from build123d import *

# Parameters (mm, degrees)
F0_W     = 431.8
F0_H     = 431.8
F1_DEPTH = 19.05
F3_DEPTH = 19.051
F5_DEPTH = 19.05
F7_DEPTH = 19.051
F9_DEPTH = 19.05


with BuildPart() as f1:
    # F0 (on Front) → F1 (new body)
    with BuildSketch(Plane.XZ):
        with Locations((215.9, 215.9)):
            Rectangle(F0_W, F0_H)
    extrude(amount=F1_DEPTH)

    # F2 (on face) → F3 (cut, through all)
    with BuildSketch(Plane.XZ.offset(19.05)):
        Polygon((177.8, 215.9), (50.8, 381), (50.8, 50.8), align=None)
        Polygon((381, 50.8), (381, 381), (254, 215.9), align=None)
    extrude(amount=-F3_DEPTH, mode=Mode.SUBTRACT)

    # F4 (on face) → F5 (join, through all)
    with BuildSketch(Plane.XZ.offset(19.05)):
        Polygon((0, 0), (0, 431.8), (-101.6, 914.4), (-152.4, 914.4), (-152.4, 0), align=None)
    extrude(amount=-F5_DEPTH)

    # F6 (on face) → F7 (cut, through all)
    with BuildSketch(Plane.XZ.offset(19.05)):
        Polygon((-101.6, 0), (-152.4, 914.4), (-152.4, 0), align=None)
    extrude(amount=-F7_DEPTH, mode=Mode.SUBTRACT)

    # F8 (on face) → F9 (join)
    with BuildSketch(Plane.XZ.offset(19.05)):
        Polygon((419.768421, 609.6), (-37.431579, 609.6), (0, 431.8), (101.6, 533.4), (343.568421, 533.4), align=None)
    extrude(amount=-F9_DEPTH)


solid = f1.part
Read the model definition and answer for the solid it produces. Units are mm, in the model's axes. A direction names the side the tool comes from. Give positions to 0.01 mm unless a question says otherwise; leave off trailing zeros. Write each loop counter-clockwise with the first axis right and the second up, starting at its lowest first coordinate (ties: lowest second). Pieces come first, ordered by that corner, then holes. Notation, with made-up numbers: (-14, -3.5) - (17, -3.5) arc R17 cw to (17, 24.5) - close; hole circle Ø2 at (15.5, 18). An arc over 180 degrees is marked (long way). Answer in a Markdown table with one row per item. Add a question column.
Item 1: Find the intervals of material crossed by L1, parallel to Z at x = 224, y = -17.25; L2, parallel to Z at x = 129, y = -15; L3, parallel to X at y = -12.25, z = 225, in increasing order.
Item 2: Section A-A, the plane x = 115.5 is taken. Write down the section's boundary in (y, z).
Item 3: Section D-D, the plane x = 13.5 is taken. Write down the section's boundary in (y, z).
Item 4: Determine the mould class of faces 1 (the face through (213, -9, 431.8)), 2 (the face through (115.19, -9.66, 297.29)), 3 (the face through (318.39, -9.66, 299.61)), 4 (the face through (50.1, -9.7, 481.9)) for opening direction X: pulls with the +X half, pulls with the -X half, needs draft (parallel to the pull), parting line crosses it, or undercut.
Item 5: A tool of negligible diameter and unlimited length cuts with its end or side. For faces 5 (the face through (316.61, -9.66, 134.51)), 6 (the face through (194, -10, 609.6)), 7 (the face through (381.14, -9.66, 570.97)), from which of +Z, -Z, +X, -X, +Y, -Y can it reach the whole face along a straight path? Write none if from no direction.
Item 6: Flat-ended cylindrical pins translate along their axes: P1, Ø5, axis at x = 320.5, z = 371.5, coming from the +Y side; P2, Ø1.5, axis at y = -2.5, z = 477, coming from the +X side; P3, Ø1.5, axis at y = -14, z = 570, coming from the -X side; P4, Ø8, axis at y = -4, z = 619.5, coming from the -X side. Find the tip coordinate at first contact, or state that the pin passes through.
Item 7: Section C-C, the plane z = 132.5 is taken. Write down the section's boundary in (x, y).
Item 8: Section B-B, the plane y = -15.75 is taken. Write down the section's boundary in (x, z).
Recorded:
| question | item | result |
|---|---|---|
| 1 | L1 | z = 0 to 431.8, 533.4 to 609.6 |
| 1 | L2 | z = 0 to 152.46, 279.34 to 431.8, 533.4 to 609.6 |
| 1 | L3 | x = -114.1 to 50.8, 170.8 to 261, 381 to 431.8 |
| 2 | outline | (-19.05, 0) - (0, 0) - (0, 134.91) - (-19.05, 134.91) - close; (-19.05, 296.89) - (0, 296.89) - (0, 431.8) - (-19.05, 431.8) - close; (-19.05, 533.4) - (0, 533.4) - (0, 609.6) - (-19.05, 609.6) - close |
| 3 | outline | (-19.05, 0) - (0, 0) - (0, 431.8) - (-19.05, 431.8) - close; (-19.05, 445.3) - (0, 445.3) - (0, 609.6) - (-19.05, 609.6) - close |
| 4 | face 1 | needs draft |
| 4 | face 2 | undercut |
| 4 | face 3 | undercut |
| 4 | face 4 | pulls with the +X half |
| 5 | face 5 | +Y, -Y |
| 5 | face 6 | +Z, +X, +Y, -Y |
| 5 | face 7 | +X, +Y, -Y |
| 6 | P1 | stops at y = 0 |
| 6 | P2 | stops at x = 45.95 |
| 6 | P3 | stops at x = -133.31 |
| 6 | P4 | stops at x = -136.24 |
| 7 | outline | (-108.96, -19.05) - (50.8, -19.05) - (50.8, 0) - (-108.96, 0) - close; (113.65, -19.05) - (318.15, -19.05) - (318.15, 0) - (113.65, 0) - close; (381, -19.05) - (431.8, -19.05) - (431.8, 0) - (381, 0) - close |
| 8 | outline | (-152.4, 914.4) - (-101.6, 0) - (431.8, 0) - (431.8, 431.8) - (0, 431.8) - (101.6, 533.4) - (343.57, 533.4) - (419.77, 609.6) - (-37.43, 609.6) - (-101.6, 914.4) - close; hole (50.8, 50.8) - (177.8, 215.9) - (50.8, 381) - close; hole (254, 215.9) - (381, 50.8) - (381, 381) - close |
